Design review of the part built by this model. Coordinates are the model's own, in mm. A direction names the side the tool comes from. Give positions to 0.01 mm unless a question says otherwise; leave off trailing zeros. Order: outer loops, then holes, each group sorted by start corner. A loop starts at its lowest first (then second) coordinate and runs counter-clockwise, first axis right, second up. Notation, with made-up numbers: (62.25, -38.75) -> (85.25, -38.75) arc R11 ccw to (85.25, -30.75) -> close; hole circle Ø8 at (3.5, 80). An arc over 180 degrees is marked (long way). Answer in a Markdown table with one row per item. Add a question column.
```python
from build123d import *

# Parameters (mm, degrees)
F0_W      = 2160
F0_H      = 1200
F1_DEPTH  = 100
F2_R      = 200
F3_R      = 200
F5_DEPTH  = 100
F6_R      = 430
F7_DEPTH  = 460
F8_W      = 100
F8_H      = 476.0843142867
F9_DEPTH  = 100
F12_DEPTH = 1200
F13_W     = 750
F13_H     = 370
F14_DEPTH = 1200.0010001
F15_R     = 330
F16_DEPTH = 560
F20_DEPTH = 100
F21_DEPTH = 1200.001
F18_R     = 320
F22_DEPTH = 680
F23_R     = 220
F24_DEPTH = 480
F26_R     = 130
F27_DEPTH = 170
F28_R     = 80
F29_DEPTH = 260
F30_R     = 140
F31_DEPTH = 200.0010001
F34_DEPTH = 50
F35_DEPTH = 50


with BuildPart() as f1:
    # F0 (on Top) → F1 (new body)
    with BuildSketch(Plane.XY):
        Rectangle(F0_W, F0_H)
    extrude(amount=F1_DEPTH)

    # F2
    f2_edges = [f1.edges().sort_by_distance(p)[0] for p in [
        (-1080, -600, 50),
    ]]
    fillet(f2_edges, radius=F2_R)

    # F3
    f3_edges = [f1.edges().sort_by_distance(p)[0] for p in [
        (1080, -600, 50),
    ]]
    fillet(f3_edges, radius=F3_R)

    # F4 (on face) → F5 (cut)
    with BuildSketch(Plane.XY.offset(100)):
        with BuildLine():
            Line((980, -400), (880, -400))
            Line((880, -400), (880, -500))
            ThreePointArc((880, -500), (950.7106781187, -470.7106781187), (980, -400))
        make_face()
        with BuildLine():
            ThreePointArc((980, -400), (880, -300), (780, -400))
            Line((780, -400), (880, -400))
            Line((880, -400), (980, -400))
        make_face()
        with BuildLine():
            Line((880, -400), (780, -400))
            ThreePointArc((780, -400), (809.2893218813, -470.7106781187), (880, -500))
            Line((880, -500), (880, -400))
        make_face()
        with BuildLine():
            Line((-880, -400), (-879.7925103978, -300.0002152599))
            ThreePointArc((-879.7925103978, -300.0002152599), (-950.6372813739, -329.2160012424), (-980, -400))
            Line((-980, -400), (-880, -400))
        make_face()
        with BuildLine():
            ThreePointArc((-780, -400), (-809.2160012424, -329.3627186261), (-879.7925103978, -300.0002152599))
            Line((-879.7925103978, -300.0002152599), (-880, -400))
            Line((-880, -400), (-780, -400))
        make_face()
        with BuildLine():
            ThreePointArc((-880, -500), (-809.2893218813, -470.7106781187), (-780, -400))
            Line((-780, -400), (-880, -400))
            Line((-880, -400), (-880, -500))
        make_face()
        with BuildLine():
            Line((-880, -400), (-980, -400))
            ThreePointArc((-980, -400), (-950.7106781187, -470.7106781187), (-880, -500))
            Line((-880, -500), (-880, -400))
        make_face()
        with BuildLine():
            ThreePointArc((-878.9625519891, 99.9989237005), (-808.117781013, 129.214709683), (-778.7550623869, 199.9987084406))
            ThreePointArc((-778.7550623869, 199.9987084406), (-949.3923437608, 270.7827071981), (-878.9625519891, 99.9989237005))
        make_face()
    extrude(amount=-F5_DEPTH, mode=Mode.SUBTRACT)

    # F6 (on face) → F7 (join)
    with BuildSketch(Plane.XY.offset(100)):
        with Locations((-318.6193108559, -39.595939219)):
            Circle(F6_R)
    extrude(amount=F7_DEPTH)

    # F8 (on face) → F9 (cut)
    with BuildSketch(Plane.XY.offset(560)):
        with Locations((-368.6193108559, -277.6380963624)):
            Rectangle(F8_W, F8_H)
        Polygon((-418.6193108559, -39.595939219), (-318.6193108559, -39.595939219), (-218.6193108559, -39.595939219), (-218.6193108559, 463.2783532143), (-418.6193108559, 463.2783532143), align=None)
        with Locations((-268.6193108559, -277.6380963624)):
            Rectangle(F8_W, F8_H)
    extrude(amount=-F9_DEPTH, mode=Mode.SUBTRACT)

    # F11 (on offset) → F12 (join)
    with BuildSketch(Plane.XZ.offset(600)):
        with BuildLine():
            ThreePointArc((40.5883862803, 0), (-64.8531724926, 254.5584412272), (-319.4116137197, 360))
            ThreePointArc((-319.4116137197, 360), (-573.9700549469, -254.5584412272), (40.5883862803, 0))
        make_face()
        with BuildLine():
            ThreePointArc((-59.4116137197, 0), (-503.2593768282, -183.8477631085), (-319.4116137197, 260))
            ThreePointArc((-319.4116137197, 260), (-135.5638506112, 183.8477631085), (-59.4116137197, 0))
        make_face(mode=Mode.SUBTRACT)
    extrude(amount=-F12_DEPTH)

    # F13 (on face) → F14 (cut, through all)
    with BuildSketch(Plane.XZ.offset(600)):
        with Locations((-321.4434087276, -185)):
            Rectangle(F13_W, F13_H)
    extrude(amount=-F14_DEPTH, mode=Mode.SUBTRACT)

    # F15 (on face) → F16 (cut)
    with BuildSketch(Plane.XY.offset(560)):
        with Locations((-318.6193108559, -39.595939219)):
            Circle(F15_R)
    extrude(amount=-F16_DEPTH, mode=Mode.SUBTRACT)

    # F19 (on offset) → F20 (join)
    with BuildSketch(Plane.XZ.offset(-600)):
        Polygon((1080.9426307678, 752.3837089539), (719.1615700722, 1278.3174514771), (-1078.9614915848, 99.5009914041), (1080.9426307678, 99.5009914041), align=None)
    extrude(amount=F20_DEPTH)

    # F11 (on offset) → F21 (cut, through all)
    with BuildSketch(Plane.XZ.offset(600)):
        with BuildLine():
            ThreePointArc((-59.4116137197, 0), (-135.5638506112, 183.8477631085), (-319.4116137197, 260))
            ThreePointArc((-319.4116137197, 260), (-503.2593768282, -183.8477631085), (-59.4116137197, 0))
        make_face()
    extrude(amount=-F21_DEPTH, mode=Mode.SUBTRACT)

    # F18 (on offset) → F22 (join)
    with BuildSketch(Plane.XZ.offset(-600)):
        with Locations((881.6419839859, 1001.6332864761)):
            Circle(F18_R)
    extrude(amount=F22_DEPTH)

    # F23 (on face) → F24 (cut)
    with BuildSketch(Plane.XZ.offset(80)):
        with Locations((881.6419839859, 1001.6332864761)):
            Circle(F23_R)
    extrude(amount=-F24_DEPTH, mode=Mode.SUBTRACT)

    # F26 (on offset) → F27 (join)
    with BuildSketch(Plane.XY.offset(1460)):
        with Locations((878.4069418907, 199.221804738)):
            Circle(F26_R)
    extrude(amount=-F27_DEPTH)

    # F28 (on face) → F29 (cut)
    with BuildSketch(Plane.XY.offset(1460)):
        with Locations((878.4069418907, 199.221804738)):
            Circle(F28_R)
    extrude(amount=-F29_DEPTH, mode=Mode.SUBTRACT)

    # F30 (on face) → F31 (cut, through all)
    with BuildSketch(Plane.XZ.offset(-400)):
        with Locations((881.6419839859, 1001.6332864761)):
            Circle(F30_R)
    extrude(amount=-F31_DEPTH, mode=Mode.SUBTRACT)

    # F33 (on offset) → F34 (join)
    with BuildSketch(Plane.YZ.offset(880)):
        Polygon((502.2943615913, 684.2531561852), (24.5764162391, 680.1151633263), (502.2943615913, 200.7880210876), align=None)
    extrude(amount=F34_DEPTH)

    # F33 (on offset) → F35 (join)
    with BuildSketch(Plane.YZ.offset(880)):
        Polygon((502.2943615913, 684.2531561852), (24.5764162391, 680.1151633263), (502.2943615913, 200.7880210876), align=None)
    extrude(amount=-F35_DEPTH)


solid = f1.part
```
1) Add section A-A, the plane y = 354.5. Write out the cut boundary in (x, z).
2) Mouldability with a two-part tool opening along Y and no side actions: class faces 1 (the face through (1080.943, 551, 421)), 2 (the face through (-390.16, -361.75, 283.92)), 3 (the face through (806, -80, 793)), 4 (the face through (-635.547, 251.018, 326.78)) as +Y half, -Y half, draft (parallel to the pull), parting line (faces both ways), or undercut.
3) Machinability: for faces 5 (the face through (930, 312, 500)), 6 (the face through (1080, 93, 49)), 7 (the face through (-320, -411, 460)), 8 (the face through (879, 400, 858)), which of the approach directions +Z, -Z, +X, -X, +Y, -Y give a long, thin tool a straight path to every point of the face, cutting with its end or side? Answer none if there is none.
4) Clearance check with flat-ended pins moving along their axes: P1, Ø12, axis at x = 854, z = 654.5, coming from the -Y side; P2, Ø1, axis at y = 126, z = 636.5, coming from the +X side; P3, Ø3, axis at x = -587, z = 362, coming from the -Y side; P4, Ø12, axis at x = 960, y = -111, coming from the -Z side. State where each tip first meets the part, or that it passes through.
5) Add section D-D, the plane z = 509. Write out the cut boundary in (x, y), and give its area (3 significant figures).
6) Add section C-C, the plane y = -162.5. Write out the cut boundary in (x, z), and give its area (3 significant figures).
7) Add section B-B, the plane z = 962. Write out the cut boundary in (x, y).
8) For L1, parallel to Z at x = 829, y = 378.5; L2, parallel to Z at x = 156.5, y = 348.5; L3, parallel to Z at x = -715.5, y = -198, list the stretches that pass through material, from the lowest coordinate up.
Verdict:
| question | item | result |
|---|---|---|
| 1 | outline | (-1080, 0) -> (-579.41, 0) arc R260 cw to (-59.41, 0) -> (1080, 0) -> (1080, 100) -> (26.42, 100) arc R360 ccw to (-146.61, 315.81) -> (-146.61, 560) -> (-218.62, 560) -> (-218.62, 460) -> (-418.62, 460) -> (-418.62, 560) -> (-490.63, 560) -> (-490.63, 316.68) arc R360 ccw to (-665.24, 100) -> (-1080, 100) -> close; (830, 349.08) -> (930, 349.08) -> (930, 682.97) -> (910.89, 682.97) arc R320 ccw (long way) to (852.39, 682.97) -> (830, 682.97) -> close; hole circle Ø440 at (881.64, 1001.63) |
| 2 | face 1 | draft |
| 2 | face 2 | undercut |
| 2 | face 3 | -Y half |
| 2 | face 4 | undercut |
| 3 | face 5 | +X, -Y |
| 3 | face 6 | -Z, +X, +Y, -Y |
| 3 | face 7 | +Z, -Y |
| 3 | face 8 | -Y |
| 4 | P1 | stops at y = 44.13 |
| 4 | P2 | stops at x = 930 |
| 4 | P3 | stops at y = -376.75 |
| 4 | P4 | stops at z = 0 |
| 5 | outline | (-454.33, 500) -> (830, 500) -> (830, 195.12) -> (930, 195.12) -> (930, 500) -> (1080.94, 500) -> (1080.94, 600) -> (-454.33, 600) -> close; (-418.62, -457.81) -> (-418.62, -354.08) arc R330 cw to (-418.62, 274.89) -> (-418.62, 378.61) arc R430 ccw to start; (-218.62, -457.81) arc R430 ccw to (-218.62, 378.61) -> (-218.62, 274.89) arc R330 cw to (-218.62, -354.08) -> close |
| 5 | area | 382,000 mm2 |
| 6 | outline | (-1080, 0) -> (-624.88, 0) -> (-624.88, 560) -> (-730.68, 560) -> (-730.68, 100) -> (-1080, 100) -> close; (-12.36, 0) -> (1080, 0) -> (1080, 100) -> (93.44, 100) -> (93.44, 560) -> (-12.36, 560) -> close |
| 6 | area | 252,000 mm2 |
| 7 | outline | (236.66, 500) -> (564.11, 500) -> (564.11, -80) -> (665.24, -80) -> (665.24, 400) -> (747.37, 400) -> (747.37, 600) -> (236.66, 600) -> close; (1015.91, 400) -> (1098.04, 400) -> (1098.04, -80) -> (1199.18, -80) -> (1199.18, 600) -> (1015.91, 600) -> close |
| 8 | L1 | z = 0 to 100, 685.99 to 788.02, 1215.24 to 1317.27 |
| 8 | L2 | z = 0 to 100 |
| 8 | L3 | z = 0 to 560 |
